Here's how the part is built. I have some questions about the finished solid (model axes, mm). A direction names the side the tool comes from. Round coordinates to 2 decimals unless told otherwise and drop trailing zeros. Write each loop counter-clockwise with the first axis right and the second up, starting at its lowest first coordinate (ties: lowest second). Pieces come first, ordered by that corner, then holes. Notation, with made-up numbers: (-22.75, 19.5) -> (20.25, 19.5) arc R26 ccw to (20.25, 39.5) -> close; hole circle Ø10 at (-20.75, -12.75). An arc over 180 degrees is marked (long way). Answer as CSV lines item,"result".
Autodesk Inventor part; units mm, degrees
ref_plane "p_to_b_XY" through (0, 0, 0) normal (0, 1, 0) x (1, 0, 0)
ref_plane "p_to_b_YZ" through (0, 0, 0) normal (1, 0, 0) x (0, 0, -1)
ref_plane "p_to_b_ZX" through (0, 0, 0) normal (0, 0, -1) x (0, 1, 0)
sketch "Sketch_10" plane through (0, 0, 0) normal (0, 0, 1) x (1, 0, 0)
  line L0 (-16, 40) -> (-16, 31)
  line L1 (-16, 31) -> (-4.899, 31)
  arc A0 (4.899, 31) -> (-4.899, 31) centre (0, 30) ccw
  line L2 (4.899, 31) -> (16, 31)
  line L3 (16, 31) -> (16, 40)
  line L4 (16, 40) -> (-16, 40)
extrude "Extrusion1" add sketch "Sketch_10" along normal mid plane 12
sketch "Sketch2" plane through (-16, 40, 6) normal (0, 1, 0) x (1, 0, 0)
  point P0 (26, 6)
hole "Hole1" at (10, 40, 0) direction (0, -1, 0) diameter 4.5 depth 9 counterbore diameter 8 counterbore depth 4.5
sketch "Sketch3" plane through (-16, 40, 6) normal (0, 1, 0) x (1, 0, 0)
  point P0 (6, 6)
hole "Hole2" at (-10, 40, 0) direction (0, -1, 0) diameter 4.5 depth 9 counterbore diameter 8 counterbore depth 4.5
ref_plane "p_to_b_XY" through (0, 0, 0) normal (0, 1, 0) x (1, 0, 0)
ref_plane "p_to_b_YZ" through (0, 0, 0) normal (1, 0, 0) x (0, 0, -1)
ref_plane "p_to_b_ZX" through (0, 0, 0) normal (0, 0, -1) x (0, 1, 0)
properties part number "SHZA10-30_p"
1. Suppose I cut it at C-C on x = -10. Please give me the cut outline in (y, z), and give its area (4 significant figures).
Numbers:
outline,"(31, -6) -> (40, -6) -> (40, -4) -> (35.5, -4) -> (35.5, -2.25) -> (31, -2.25) -> close; (31, 2.25) -> (35.5, 2.25) -> (35.5, 4) -> (40, 4) -> (40, 6) -> (31, 6) -> close"
area,"51.75 mm^2"
2. If we mould it in two halves opening along Z, with no side actions, what happens to faces 1 (the face through (-11.897, 33.218, 1.21)), 2 (the face through (0, 35, 0)), 3 (the face through (0, 36, 6))? For each: released by +Z, released by -Z, zero draft, split by the parting line, or undercut.
Numbers:
face 1,"undercut"
face 2,"zero draft"
face 3,"released by +Z"
3. For pin 1 Ø4 at (x, z) = (-10, -0.5) entering from +Y, with a flat end and sliding along its axis, tell me the tip position at first contact or that it passes through.
Numbers:
pin 1,"stops at y = 35.5"
4. Suppose I cut it at D-D on y = 39.5. Please give me the cut outline in (x, z), and give its area (3 significant figures).
Numbers:
outline,"(-16, -6) -> (16, -6) -> (16, 6) -> (-16, 6) -> close; hole circle Ø8 at (-10, 0); hole circle Ø8 at (10, 0)"
area,"283 mm^2"
5. If I drill on line 1 (Z direction, x = -10, y = 36.65); line 2 (X direction, y = 38.05, z = 0); line 3 (Z direction, x = 10, y = 32.5), over which ranges is the centre line in solid material (lowest first)?
Numbers:
line 1,"z = -6 to -4, 4 to 6"
line 2,"x = -16 to -14, -6 to 6, 14 to 16"
line 3,"z = -6 to -2.25, 2.25 to 6"
6. Suppose I cut it at A-A on z = 0. Please give me the cut outline in (x, y), and give its area (3 significant figures).
Numbers:
outline,"(-16, 31) -> (-12.25, 31) -> (-12.25, 35.5) -> (-14, 35.5) -> (-14, 40) -> (-16, 40) -> close; (-7.75, 31) -> (-4.9, 31) arc R5 cw to (4.9, 31) -> (7.75, 31) -> (7.75, 35.5) -> (6, 35.5) -> (6, 40) -> (-6, 40) -> (-6, 35.5) -> (-7.75, 35.5) -> close; (12.25, 31) -> (16, 31) -> (16, 40) -> (14, 40) -> (14, 35.5) -> (12.25, 35.5) -> close"
area,"146 mm^2"
7. Suppose I cut it at B-B on y = 33. Please give me the cut outline in (x, z), and give its area (3 significant figures).
Numbers:
outline,"(-16, -6) -> (-4, -6) -> (-4, 6) -> (-16, 6) -> close; (4, -6) -> (16, -6) -> (16, 6) -> (4, 6) -> close; hole circle Ø4.5 at (-10, 0); hole circle Ø4.5 at (10, 0)"
area,"256 mm^2"
8. On a 3-axis mill with a long thin cutter (end or side, diameter ignored), from which of +Z, -Z, +X, -X, +Y, -Y can I reach the whole of each face in a straight line? I mean faces 4 (the face through (12, 35.5, 2)), 5 (the face through (0, 40, 0)). Say none if no direction works.
Numbers:
face 4,"+Y"
face 5,"+Z, -Z, +X, -X, +Y"
